For this review, take the finished solid that the model builds, in its own axes (mm). Coordinates: 2 decimals unless noted, no trailing zeros. Write each loop counter-clockwise with the first axis right and the second up, starting at its lowest first coordinate (ties: lowest second). Pieces come first, ordered by that corner, then holes. Notation, with made-up numbers: M 76,-26.5 L 133,-26.5 A29 ccw 133,0.5 Z; hole C 33,14 d1. An arc over 180 degrees is marked long. Return JSON: item names as keys, results as strings.
```python
from build123d import *

# Parameters (mm, degrees)
SKETCH1_W               = 35
SKETCH1_H               = 20
BOSS_EXTRUDE1_DEPTH     = 40
CUT_EXTRUDE1_DEPTH      = 40
CUT_EXTRUDE2_DEPTH      = 45.791182168
CUT_EXTRUDE2_DEPTH_BACK = 45.791182168
SKETCH6_R               = 2
CUT_EXTRUDE3_DEPTH      = 45.791182168


with BuildPart() as part:
    # Sketch1 → Boss-Extrude1 (new body)
    with BuildSketch(Plane.XY):
        Rectangle(SKETCH1_W, SKETCH1_H)
    extrude(amount=BOSS_EXTRUDE1_DEPTH)

    # Sketch3 → Cut-Extrude1 (cut)
    with BuildSketch(Plane.XY.offset(40)):
        Polygon((-17.5, 10), (-17.5, 6), (0, 10), align=None)
        Polygon((17.5, 10), (0, 10), (17.5, 6), align=None)
        Polygon((17.5, -6), (0, -10), (17.5, -10), align=None)
        Polygon((0, -10), (-17.5, -6), (-17.5, -10), align=None)
    extrude(amount=-CUT_EXTRUDE1_DEPTH, mode=Mode.SUBTRACT)

    # Sketch5 → Cut-Extrude2 (cut, two sides: drawn at the far end of the back side and taken through both)
    with BuildSketch(Plane(origin=(0, 0, 0), x_dir=(1, 0, 0), z_dir=(0, 1, 0)).offset(-CUT_EXTRUDE2_DEPTH_BACK)):
        Polygon((-17.5, 0), (0, 0), (-17.5, -6), align=None)
        Polygon((17.5, -6), (17.5, 0), (0, 0), align=None)
        Polygon((17.5, -40), (0, -40), (17.5, -34), align=None)
        Polygon((-17.5, -40), (-17.5, -34), (0, -40), align=None)
    extrude(amount=CUT_EXTRUDE2_DEPTH + CUT_EXTRUDE2_DEPTH_BACK, mode=Mode.SUBTRACT)

    # Sketch6 → Cut-Extrude3 (cut, through all)
    with BuildSketch(Plane.XY):
        with Locations(Location((-14.5, 0, 0), (0, 0, 180))):
            Circle(SKETCH6_R)
        with Locations(Location((14.5, 0, 0), (0, 0, 180))):
            Circle(SKETCH6_R)
    extrude(amount=CUT_EXTRUDE3_DEPTH, mode=Mode.SUBTRACT)


solid = part.part
```
1. We need section C-C (y = -2.5). State the section outline as (x, z) points, plus the area to 3 significant figures.
Checks:
{"outline": "M -17.5,6 L 0,0 L 17.5,6 L 17.5,34 L 0,40 L -17.5,34 Z", "area": "1,190 mm2"}
2. Clearance check with flat-ended pins moving along their axes: pin 1 Ø12 at (x, y) = (0, 0) entering from +Z; pin 2 Ø4 at (x, z) = (-1, 28) entering from +Y; pin 3 Ø12 at (x, y) = (9, 1.5) entering from +Z. State where each tip first meets the part, or that it passes through.
Checks:
{"pin 1": "z = 40", "pin 2": "y = 10", "pin 3": "z = 38.97"}
3. We need section B-B (x = -14.5). State the section outline as (y, z) points.
Checks:
{"outline": "M -6.69,4.97 L -2,4.97 L -2,35.03 L -6.69,35.03 Z; M 2,4.97 L 6.69,4.97 L 6.69,35.03 L 2,35.03 Z"}
4. We need section D-D (y = 0.75). State the section outline as (x, z) points, plus the area to 3 significant figures.
Checks:
{"outline": "M -17.5,6 L -16.35,5.61 L -16.35,34.39 L -17.5,34 Z; M -12.65,4.34 L 0,0 L 12.65,4.34 L 12.65,35.66 L 0,40 L -12.65,35.66 Z; M 16.35,5.61 L 17.5,6 L 17.5,34 L 16.35,34.39 Z", "area": "967 mm2"}
5. Wall thickness on L1, parallel to Y at x = -14.5, z = 28.5; L2, parallel to Y at x = -14, z = 20; L3, parallel to Z at x = -5, y = -1: over which ranges is each line inside the solid? List them lowest first. Write a range as from..to.
Checks:
{"L1": "-6.69..-2, 2..6.69", "L2": "-6.8..-1.94, 1.94..6.8", "L3": "1.71..38.29"}
6. We need section A-A (z = 8.5). State the section outline as (x, y) points, plus the area to 3 significant figures.
Checks:
{"outline": "M -17.5,-6 L 0,-10 L 17.5,-6 L 17.5,6 L 0,10 L -17.5,6 Z; hole C -14.5,0 d4; hole C 14.5,0 d4", "area": "535 mm2"}
